Design review of the part built by this model. Coordinates are the model's own, in mm. Give positions to 0.01 mm unless a question says otherwise; leave off trailing zeros. Order: outer loops, then holes, each group sorted by start corner. A loop starts at its lowest first (then second) coordinate and runs counter-clockwise, first axis right, second up.
```python
from build123d import *

# Parameters (mm, degrees)
BOSS_EXTRUDE1_DEPTH            = 550
SKETCH2_W                      = 46
SKETCH2_H                      = 10
CUT_EXTRUDE1_DEPTH             = 35
SKETCH3_W                      = 46
SKETCH3_H                      = 10
CUT_EXTRUDE2_DEPTH             = 35
F_3_0MM_DOWEL_HOLE1_AT_2_COUNT = 2
F_3_0MM_DOWEL_HOLE1_AT_2_PITCH = 12
F_3_0MM_DOWEL_HOLE1_AT_3_COUNT = 2
F_3_0MM_DOWEL_HOLE1_AT_3_PITCH = 23.323807579
F_3_0MM_DOWEL_HOLE1_AT_4_COUNT = 2
F_3_0MM_DOWEL_HOLE1_AT_4_PITCH = 20
F_3_0MM_DOWEL_HOLE2_AT_2_COUNT = 2
F_3_0MM_DOWEL_HOLE2_AT_2_PITCH = 14
F_3_0MM_DOWEL_HOLE3_AT_2_COUNT = 2
F_3_0MM_DOWEL_HOLE3_AT_2_PITCH = 15
F_3_0MM_DOWEL_HOLE3_AT_3_COUNT = 2
F_3_0MM_DOWEL_HOLE3_AT_3_PITCH = 75
F_3_0MM_DOWEL_HOLE3_AT_4_COUNT = 2
F_3_0MM_DOWEL_HOLE3_AT_4_PITCH = 90
F_3_0MM_DOWEL_HOLE3_AT_5_COUNT = 2
F_3_0MM_DOWEL_HOLE3_AT_5_PITCH = 150
F_3_0MM_DOWEL_HOLE3_AT_6_COUNT = 2
F_3_0MM_DOWEL_HOLE3_AT_6_PITCH = 165


with BuildPart() as part:
    # Sketch1 → Boss-Extrude1 (new body)
    with BuildSketch(Plane.XY):
        Polygon((-2.128855562, -13.394137553), (1.871144438, -13.394137553), (1.871144438, -2.394137553), (31.871144438, -2.394137553), (31.871144438, 1.605862447), (1.871144438, 1.605862447), (1.871144438, 11.605862447), (-2.128855562, 11.605862447), align=None)
    extrude(amount=BOSS_EXTRUDE1_DEPTH)

    # Sketch2 → Cut-Extrude1 (cut, through all)
    with BuildSketch(Plane.ZY.offset(2.128855562)):
        with Locations((23, 6.605862447)):
            Rectangle(SKETCH2_W, SKETCH2_H)
    cut_extrude1 = extrude(amount=-CUT_EXTRUDE1_DEPTH, mode=Mode.SUBTRACT)

    # Sketch3 → Cut-Extrude2 (cut, through all)
    with BuildSketch(Plane.ZY.offset(2.128855562)):
        with Locations((275, 6.605862447)):
            Rectangle(SKETCH3_W, SKETCH3_H)
    extrude(amount=-CUT_EXTRUDE2_DEPTH, mode=Mode.SUBTRACT)

    # Sketch6 → Ø3.0mm Dowel Hole1 (revolve, cut)
    with BuildSketch(Plane(origin=(17.871144438, 1.605862447, 13), x_dir=(0, 0, 1), z_dir=(1, 0, 0))):
        Polygon((0, 0), (0, 15.901290929), (1.5, 15), (1.5, 0), align=None)
    f_3_0mm_dowel_hole1 = revolve(axis=Axis((17.871144438, 7.955862447, 13), (0, -1, 0)), mode=Mode.SUBTRACT)

    # Ø3.0mm Dowel Hole1 at 2: Ø3.0mm Dowel Hole1 ×2
    with Locations(*[(-i * F_3_0MM_DOWEL_HOLE1_AT_2_PITCH, 0, 0) for i in range(1, F_3_0MM_DOWEL_HOLE1_AT_2_COUNT)]):
        add(f_3_0mm_dowel_hole1, mode=Mode.SUBTRACT)

    # Ø3.0mm Dowel Hole1 at 3: Ø3.0mm Dowel Hole1 ×2
    with Locations(*[Vector(-0.514495755, 0, 0.857492926) * (i * F_3_0MM_DOWEL_HOLE1_AT_3_PITCH) for i in range(1, F_3_0MM_DOWEL_HOLE1_AT_3_COUNT)]):
        add(f_3_0mm_dowel_hole1, mode=Mode.SUBTRACT)

    # Ø3.0mm Dowel Hole1 at 4: Ø3.0mm Dowel Hole1 ×2
    with Locations(*[(0, 0, i * F_3_0MM_DOWEL_HOLE1_AT_4_PITCH) for i in range(1, F_3_0MM_DOWEL_HOLE1_AT_4_COUNT)]):
        add(f_3_0mm_dowel_hole1, mode=Mode.SUBTRACT)

    # Mirror2: Cut-Extrude1, Ø3.0mm Dowel Hole1 across plane
    add(cut_extrude1.mirror(Plane.XY.offset(275)), mode=Mode.SUBTRACT)
    add(f_3_0mm_dowel_hole1.mirror(Plane.XY.offset(275)), mode=Mode.SUBTRACT)

    # Mirror2 copy 1 sketch → Mirror2 copy 1 (revolve, cut)
    with BuildSketch(Plane(origin=(5.871144438, 1.605862447, 537), x_dir=(0, 0, -1), z_dir=(1, 0, 0))):
        Polygon((0, 0), (0, -15.901290929), (1.5, -15), (1.5, 0), align=None)
    revolve(axis=Axis((5.871144438, 7.955862447, 537), (0, 1, 0)), mode=Mode.SUBTRACT)

    # Mirror2 copy 2 sketch → Mirror2 copy 2 (revolve, cut)
    with BuildSketch(Plane(origin=(5.871144438, 1.605862447, 517), x_dir=(0, 0, -1), z_dir=(1, 0, 0))):
        Polygon((0, 0), (0, -15.901290929), (1.5, -15), (1.5, 0), align=None)
    revolve(axis=Axis((5.871144438, 7.955862447, 517), (0, 1, 0)), mode=Mode.SUBTRACT)

    # Mirror2 copy 3 sketch → Mirror2 copy 3 (revolve, cut)
    with BuildSketch(Plane(origin=(17.871144438, 1.605862447, 517), x_dir=(0, 0, -1), z_dir=(1, 0, 0))):
        Polygon((0, 0), (0, -15.901290929), (1.5, -15), (1.5, 0), align=None)
    revolve(axis=Axis((17.871144438, 7.955862447, 517), (0, 1, 0)), mode=Mode.SUBTRACT)

    # Sketch10 → Ø3.0mm Dowel Hole2 (revolve, cut)
    with BuildSketch(Plane(origin=(23.871144438, 1.605862447, 285), x_dir=(0, 0, 1), z_dir=(1, 0, 0))):
        Polygon((0, 0), (0, 15.901290929), (1.5, 15), (1.5, 0), align=None)
    f_3_0mm_dowel_hole2 = revolve(axis=Axis((23.871144438, 7.955862447, 285), (0, -1, 0)), mode=Mode.SUBTRACT)

    # Ø3.0mm Dowel Hole2 at 2: Ø3.0mm Dowel Hole2 ×2
    with Locations(*[(-i * F_3_0MM_DOWEL_HOLE2_AT_2_PITCH, 0, 0) for i in range(1, F_3_0MM_DOWEL_HOLE2_AT_2_COUNT)]):
        add(f_3_0mm_dowel_hole2, mode=Mode.SUBTRACT)

    # Mirror3: Ø3.0mm Dowel Hole2 across plane
    add(f_3_0mm_dowel_hole2.mirror(Plane.XY.offset(275)), mode=Mode.SUBTRACT)

    # Mirror3 copy 1 sketch → Mirror3 copy 1 (revolve, cut)
    with BuildSketch(Plane(origin=(9.871144438, 1.605862447, 265), x_dir=(0, 0, -1), z_dir=(1, 0, 0))):
        Polygon((0, 0), (0, -15.901290929), (1.5, -15), (1.5, 0), align=None)
    revolve(axis=Axis((9.871144438, 7.955862447, 265), (0, 1, 0)), mode=Mode.SUBTRACT)

    # Sketch14 → Ø3.0mm Dowel Hole3 (revolve, cut)
    with BuildSketch(Plane(origin=(16.296779724, 1.605862447, 231.5), x_dir=(0, 0, 1), z_dir=(1, 0, 0))):
        Polygon((0, 0), (0, 15.901290929), (1.5, 15), (1.5, 0), align=None)
    f_3_0mm_dowel_hole3 = revolve(axis=Axis((16.296779724, 7.955862447, 231.5), (0, -1, 0)), mode=Mode.SUBTRACT)

    # Ø3.0mm Dowel Hole3 at 2: Ø3.0mm Dowel Hole3 ×2
    with Locations(*[(0, 0, -i * F_3_0MM_DOWEL_HOLE3_AT_2_PITCH) for i in range(1, F_3_0MM_DOWEL_HOLE3_AT_2_COUNT)]):
        add(f_3_0mm_dowel_hole3, mode=Mode.SUBTRACT)

    # Ø3.0mm Dowel Hole3 at 3: Ø3.0mm Dowel Hole3 ×2
    with Locations(*[(0, 0, -i * F_3_0MM_DOWEL_HOLE3_AT_3_PITCH) for i in range(1, F_3_0MM_DOWEL_HOLE3_AT_3_COUNT)]):
        add(f_3_0mm_dowel_hole3, mode=Mode.SUBTRACT)

    # Ø3.0mm Dowel Hole3 at 4: Ø3.0mm Dowel Hole3 ×2
    with Locations(*[(0, 0, -i * F_3_0MM_DOWEL_HOLE3_AT_4_PITCH) for i in range(1, F_3_0MM_DOWEL_HOLE3_AT_4_COUNT)]):
        add(f_3_0mm_dowel_hole3, mode=Mode.SUBTRACT)

    # Ø3.0mm Dowel Hole3 at 5: Ø3.0mm Dowel Hole3 ×2
    with Locations(*[(0, 0, -i * F_3_0MM_DOWEL_HOLE3_AT_5_PITCH) for i in range(1, F_3_0MM_DOWEL_HOLE3_AT_5_COUNT)]):
        add(f_3_0mm_dowel_hole3, mode=Mode.SUBTRACT)

    # Ø3.0mm Dowel Hole3 at 6: Ø3.0mm Dowel Hole3 ×2
    with Locations(*[(0, 0, -i * F_3_0MM_DOWEL_HOLE3_AT_6_PITCH) for i in range(1, F_3_0MM_DOWEL_HOLE3_AT_6_COUNT)]):
        add(f_3_0mm_dowel_hole3, mode=Mode.SUBTRACT)

    # Mirror4: Ø3.0mm Dowel Hole3 across plane
    add(f_3_0mm_dowel_hole3.mirror(Plane.XY.offset(275)), mode=Mode.SUBTRACT)

    # Mirror4 copy 1 sketch → Mirror4 copy 1 (revolve, cut)
    with BuildSketch(Plane(origin=(16.296779724, 1.605862447, 333.5), x_dir=(0, 0, -1), z_dir=(1, 0, 0))):
        Polygon((0, 0), (0, -15.901290929), (1.5, -15), (1.5, 0), align=None)
    revolve(axis=Axis((16.296779724, 7.955862447, 333.5), (0, 1, 0)), mode=Mode.SUBTRACT)

    # Mirror4 copy 2 sketch → Mirror4 copy 2 (revolve, cut)
    with BuildSketch(Plane(origin=(16.296779724, 1.605862447, 393.5), x_dir=(0, 0, -1), z_dir=(1, 0, 0))):
        Polygon((0, 0), (0, -15.901290929), (1.5, -15), (1.5, 0), align=None)
    revolve(axis=Axis((16.296779724, 7.955862447, 393.5), (0, 1, 0)), mode=Mode.SUBTRACT)

    # Mirror4 copy 3 sketch → Mirror4 copy 3 (revolve, cut)
    with BuildSketch(Plane(origin=(16.296779724, 1.605862447, 408.5), x_dir=(0, 0, -1), z_dir=(1, 0, 0))):
        Polygon((0, 0), (0, -15.901290929), (1.5, -15), (1.5, 0), align=None)
    revolve(axis=Axis((16.296779724, 7.955862447, 408.5), (0, 1, 0)), mode=Mode.SUBTRACT)

    # Mirror4 copy 4 sketch → Mirror4 copy 4 (revolve, cut)
    with BuildSketch(Plane(origin=(16.296779724, 1.605862447, 468.5), x_dir=(0, 0, -1), z_dir=(1, 0, 0))):
        Polygon((0, 0), (0, -15.901290929), (1.5, -15), (1.5, 0), align=None)
    revolve(axis=Axis((16.296779724, 7.955862447, 468.5), (0, 1, 0)), mode=Mode.SUBTRACT)

    # Mirror4 copy 5 sketch → Mirror4 copy 5 (revolve, cut)
    with BuildSketch(Plane(origin=(16.296779724, 1.605862447, 483.5), x_dir=(0, 0, -1), z_dir=(1, 0, 0))):
        Polygon((0, 0), (0, -15.901290929), (1.5, -15), (1.5, 0), align=None)
    revolve(axis=Axis((16.296779724, 7.955862447, 483.5), (0, 1, 0)), mode=Mode.SUBTRACT)


solid = part.part
```
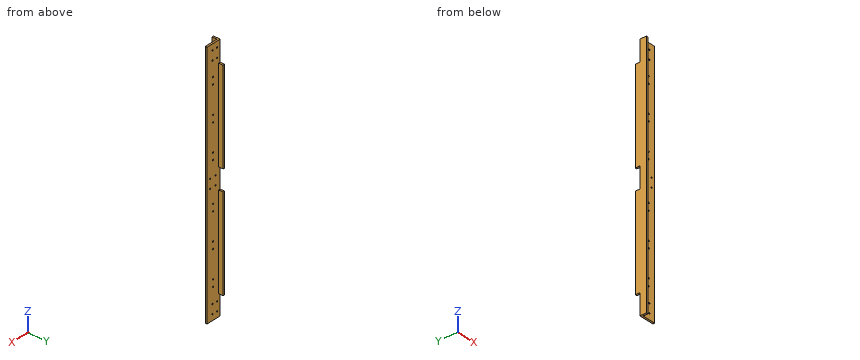
1. Take a section at A-A (z = 341). State the section outline as (x, y) points, then the cut area to 3 significant figures.
Recorded:
outline: (-2.13, -13.39) - (1.87, -13.39) - (1.87, -2.39) - (31.87, -2.39) - (31.87, 1.61) - (1.87, 1.61) - (1.87, 11.61) - (-2.13, 11.61) - close
area: 220 mm2
2. Take a section at B-B (y = -9.5). State the section outline as (x, z) points.
Recorded:
outline: (-2.13, 0) - (1.87, 0) - (1.87, 550) - (-2.13, 550) - close
3. For pin 1 (12 mm diameter, centred on x = 21.5, y = -8.5, fed in from +Z); pin 2 (5 mm diameter, centred on x = 16.3, z = 231.5, fed in from +Y); pin 3 (2 mm diameter, centred on y = 7, z = 156.5, fed in from +X); pin 4 (4 mm diameter, centred on x = 23.87, z = 265, fed in from -Y), all flat-tipped, find the tip position at first contact; note any pin that passes through.
Recorded:
pin 1: passes through
pin 2: stops at y = 1.61
pin 3: stops at x = 1.87
pin 4: stops at y = -2.39
4. For line 1 along X through (y, z) = (-0.75, 285); line 2 along X through (y, z) = (0.45, 13); line 3 along X through (y, z) = (-9.5, 150), list the stretches that pass through material, from the lowest coordinate up.
Recorded:
line 1: x = -2.13 to 8.37, 11.37 to 22.37, 25.37 to 31.87
line 2: x = -2.13 to 4.37, 7.37 to 16.37, 19.37 to 31.87
line 3: x = -2.13 to 1.87
